Autodesk Inventor part; units mm, degrees
ref_plane "YZ Plane" through (0, 0, 0) normal (1, 0, 0) x (0, 1, 0)
ref_plane "XZ Plane" through (0, 0, 0) normal (0, 1, 0) x (-1, 0, 0)
ref_plane "XY Plane" through (0, 0, 0) normal (0, 0, 1) x (1, 0, 0)
sketch "Sketch1" plane through (0, 0, 0) normal (0, 0, 1) x (1, 0, 0)
  circle A0 centre (0, 0) radius 2.75
  line L0 (0.25, -4.8394) -> (0.25, 4.8394)
  line L1 (0.25, 4.8394) -> (-0.25, 4.8394)
  line L2 (-0.25, 4.8394) -> (-0.25, -4.8394)
  line L3 (-0.25, -4.8394) -> (0.25, -4.8394)
  line L4 (0.25, -4.8394) -> (-0.25, 4.8394) construction
  line L5 (0.25, 4.8394) -> (-0.25, -4.8394) construction
  point P0 (-0.25, 2.7386)
  point P1 (-0.25, -2.7386)
  point P2 (0.25, -2.7386)
  point P3 (0.25, 2.7386)
  dimension "d0" = 5.5
  dimension "d1" = 0.5
extrude "Extrusion1" add sketch "Sketch1" along normal blind 30 contours A0 L0 | L0 A0 L2 | L2 A0
extrude "Extrusion2" cut sketch "Sketch1" along normal blind 1 contours L0 A0 L2
sketch "Sketch2" plane through (0, 0, 30) normal (0, 0, 1) x (1, 0, 0)
  circle A0 centre (0, 0) radius 3.15
  dimension "d6" = 6.3
extrude "Extrusion3" add sketch "Sketch2" against normal blind 8
thread "Thread1"
sketch "Sketch3" plane through (0, 0, 30) normal (0, 0, 1) x (1, 0, 0)
  circle A0 centre (0, 0) radius 8
  dimension "d11" = 16
extrude "Extrusion4" add sketch "Sketch3" along normal blind 10
sketch "Sketch4" plane through (0, 0, 30) normal (0, 0, -1) x (-1, 0, 0)
  line L0 (-8, 13.3929) -> (8, 13.3929)
  line L1 (8, 13.3929) -> (8, -13.3929)
  line L2 (8, -13.3929) -> (-8, -13.3929)
  line L3 (-8, -13.3929) -> (-8, 13.3929)
  line L4 (-8, 13.3929) -> (8, -13.3929) construction
  line L5 (8, 13.3929) -> (-8, -13.3929) construction
  line L6 (8, 0) -> (-8, 0)
  circle A0 centre (0, 0) radius 8
  point P0 (-5.7062, 5.6071)
  dimension "d17" = 19
extrude "Extrusion5" add sketch "Sketch4" against normal blind 1 contours A0 L1 L2 L3 | L6 A0 picked at (-1.8203, -3.4339)
properties part number "Potentiometer" material "ABS Plastic"
Could you check a few things on this model? Use its own coordinates, in mm. A direction names the side the tool comes from. Give positions to 0.01 mm unless a question says otherwise; leave off trailing zeros. Order: outer loops, then holes, each group sorted by start corner. A loop starts at its lowest first (then second) coordinate and runs counter-clockwise, first axis right, second up.
Q1. We'd pull the mould along X, two halves only. Please class faces 5 (the flat face through (-0.25, 0, 0.5)), 6 (the flat face through (-1, 0, 0)), 7 (the cylindrical face through (-0.596, 2.685, 10.846)), 8 (the flat face through (-8, -6.6, 30.5)): +X half, -X half, draft (parallel to the pull), parting line (faces both ways), or undercut.
Q2. Suppose I cut it at C-C, the plane x = -7. Write out the boundary of the cut face in (y, z).
Q3. I'm going to push flat-ended pins straight in: P1, Ø2, axis at x = 5.5, y = -9.5, coming from the +Z side; P2, Ø0.5, axis at y = 0.5, z = 0.5, coming from the -X side; P3, Ø1.1, axis at y = 0.5, z = 0.5, coming from the +X side. Where does each tip first touch, or does it pass through?
Q4. For faces 1 (the flat face through (1, 0, 0)), 2 (the cylindrical face through (-1.73, 7.81, 34.93)), 3 (the flat face through (0.25, 0, 0.5)), 4 (the cylindrical face through (-2.5, -1.917, 26.056)), which set-ups out of +Z, -Z, +X, -X, +Y, -Y let a thin tool reach every point of the face, with its end or its side?
Q5. Suppose I cut it at B-B, the plane z = 17.5. Write out the boundary of the cut face in (x, y), and give its area (3 significant figures).
Q6. Suppose I cut it at A-A, the plane y = -5.5. Write out the boundary of the cut face in (x, z), and give its area (3 significant figures).
Q7. Suppose I cut it at D-D, the plane y = 1.75. Write out the boundary of the cut face in (x, z).
Q8. If I drill on line 1 along Z through (x, y) = (-5.5, -9.25); line 2 along Y through (x, z) = (0.25, 3.5); line 3 along Z through (x, y) = (-5.25, 0.25), over which ranges is the centre line in solid material (lowest first)?
Solution:
1. face 5: undercut
1. face 6: draft
1. face 7: parting line
1. face 8: -X half
2. outline: (-13.39, 30) - (3.87, 30) - (3.87, 40) - (-3.87, 40) - (-3.87, 31) - (-13.39, 31) - close
3. P1: stops at z = 31
3. P2: stops at x = -2.74
3. P3: stops at x = 2.75
4. face 1: -Z, +X, -X, +Y, -Y
4. face 2: +Z
4. face 3: -Z, +Y, -Y
4. face 4: -Z
5. outline: circle Ø5.5 at (0, 0)
5. area: 23.8 mm2
6. outline: (-8, 30) - (8, 30) - (8, 31) - (5.81, 31) - (5.81, 40) - (-5.81, 40) - (-5.81, 31) - (-8, 31) - close
6. area: 121 mm2
7. outline: (-7.81, 30) - (-2.62, 30) - (-2.62, 22) - (-2.12, 22) - (-2.12, 0) - (-0.25, 0) - (-0.25, 1) - (0.25, 1) - (0.25, 0) - (2.12, 0) - (2.12, 22) - (2.62, 22) - (2.62, 30) - (7.81, 30) - (7.81, 40) - (-7.81, 40) - close
8. line 1: z = 30 to 31
8. line 2: y = -2.74 to 2.74
8. line 3: z = 30 to 40
